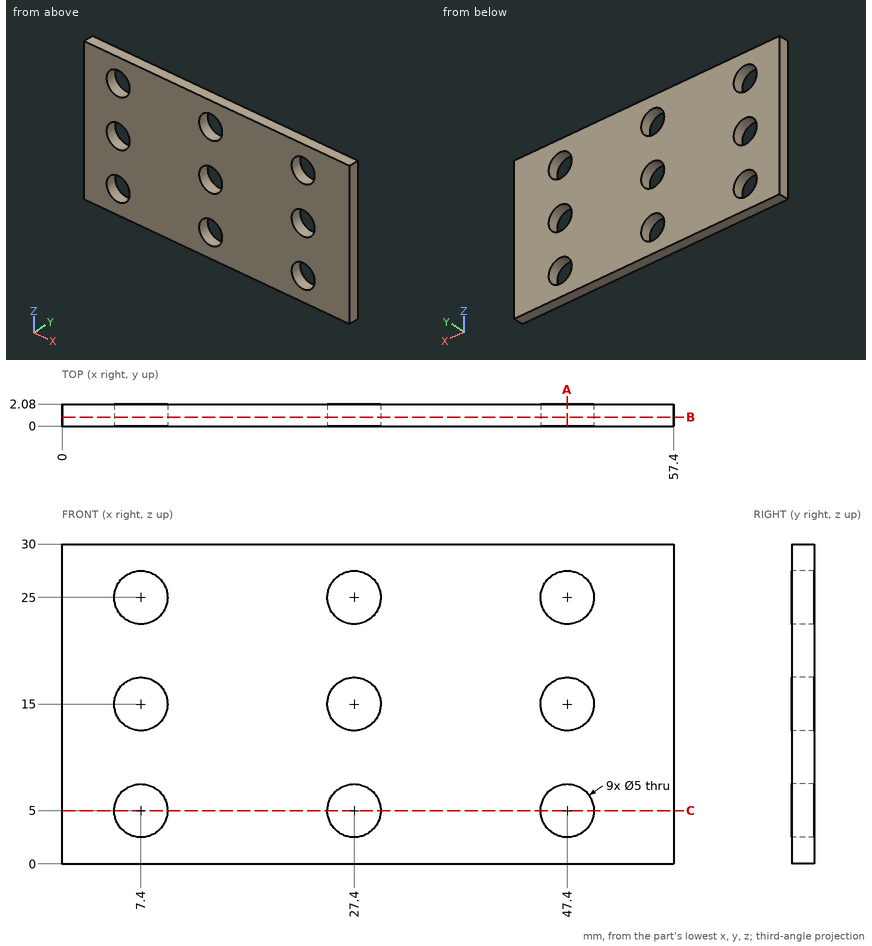
Source: three-view drawing plus pictorial views. Frame: mm from the lowest corner of the part. Coordinates: 2 decimals unless noted, no trailing zeros. Loops run counter-clockwise (first coordinate to the right, second up) from the corner with the lowest first, then second, coordinate; pieces in that order, holes last. Notation, with made-up numbers: (75.5, 66) - (87.5, 66) arc R34 ccw to (87.5, 97) - close; hole circle Ø10 at (5.5, -4.75). An arc over 180 degrees is marked (long way). One line per item, written item: value. Start each with the question number.
1. Contact query for flat-ended pins moving along their axis: P1, Ø3, axis at x = 7.4, z = 5, coming from the -Y side; P2, Ø6.5, axis at x = 7.4, z = 25, coming from the +Y side. Output: stop coordinate, or through.
2. Ray query, L1, parallel to X at y = 1.1, z = 25; L2, parallel to X at y = 1.8, z = 7; L3, parallel to Z at x = 26, y = 1.1. Return the intervals inside material, ascending.
3. Section B-B (y = 0.85). State how many separate pieces and enclosed holes the cut face has, and give its area (3 significant figures).
4. Section A-A (x = 47.4). Return the cut outline in (y, z).
5. Section C-C (z = 5). Return the cut outline in (x, y).
Verdict:
1. P1: passes through
1. P2: stops at y = 2.08
2. L1: x = 0 to 4.9, 9.9 to 24.9, 29.9 to 44.9, 49.9 to 57.4
2. L2: x = 0 to 5.9, 8.9 to 25.9, 28.9 to 45.9, 48.9 to 57.4
2. L3: z = 0 to 2.93, 7.07 to 12.93, 17.07 to 22.93, 27.07 to 30
3. separate pieces: 1
3. enclosed holes: 9
3. area: 1,550 mm2
4. outline: (0, 0) - (2.08, 0) - (2.08, 2.5) - (0, 2.5) - close; (0, 7.5) - (2.08, 7.5) - (2.08, 12.5) - (0, 12.5) - close; (0, 17.5) - (2.08, 17.5) - (2.08, 22.5) - (0, 22.5) - close; (0, 27.5) - (2.08, 27.5) - (2.08, 30) - (0, 30) - close
5. outline: (0, 0) - (4.9, 0) - (4.9, 2.08) - (0, 2.08) - close; (9.9, 0) - (24.9, 0) - (24.9, 2.08) - (9.9, 2.08) - close; (29.9, 0) - (44.9, 0) - (44.9, 2.08) - (29.9, 2.08) - close; (49.9, 0) - (57.4, 0) - (57.4, 2.08) - (49.9, 2.08) - close
